The model under review builds one solid part; all positions refer to its coordinate system, in mm. A direction names the side the tool comes from. Give positions to 0.01 mm unless a question says otherwise; leave off trailing zeros. Loops run counter-clockwise (first coordinate to the right, second up) from the corner with the lowest first, then second, coordinate; pieces in that order, holes last. Notation, with made-up numbers: M -17.5,-24.75 L 1.5,-24.75 A21 ccw 1.5,-8.75 Z; hole C 71,-16.75 d7. An arc over 180 degrees is marked long. Write item = value, one per line. Start each with the question number.
1. We need section C-C on x = 60.5. Give the boundary of the cut face in (y, z).
2. Wall thickness on line 1 along Y through (x, z) = (37, -63); line 2 along Z through (x, y) = (17, 10); line 3 along Z through (x, y) = (38, 7.25): over which ranges is each line inside the solid? List them lowest first. Write a range as from..to.
3. For faces 5 (the face through (34.194, 2.465, -49.688)), 6 (the face through (46, 0, -1)), 7 (the face through (22.761, 17.521, 51.585)), list the 3-axis set-ups (+Z, -Z, +X, -X, +Y, -Y) from which the entire face can be reached by the end or side of a thin tool; tool diameter is ignored.
4. For pin 1 (1 mm diameter, centred on x = 54, y = 12, fed in from +Z); pin 2 (6 mm diameter, centred on y = 16.5, z = -31.5, fed in from +X); pin 3 (9 mm diameter, centred on y = 10, z = -63, fed in from +X); pin 4 (8 mm diameter, centred on x = 30.82, z = 53.37, fed in from -Y), all flat-tipped, find the tip position at first contact; note any pin that passes through.
5. We need section A-A on y = 7.5. Give the boundary of the cut face in (x, z) (3 decimals).
6. Draft analysis for pull direction X (two halves, no side actions). For faces 1 (the face through (33, 16, 51)), 2 (the face through (46, 20, -1)), 3 (the face through (29, 5, 51)), 4 (the face through (74.98, 9.86, -1.65)), state which applies: pulls with the +X half, pulls with the -X half, needs draft (parallel to the pull), parting line crosses it, or undercut.
7. We need section B-B on z = 0. Give the boundary of the cut face in (x, y), then the cut area to 3 significant figures.
from build123d import *

# Parameters (mm, degrees)
BOSS_EXTRUDE1_DEPTH = 20
SKETCH2_R           = 5
CUT_EXTRUDE1_DEPTH  = 150
SKETCH3_R           = 8.25
CUT_EXTRUDE3_DEPTH  = 4
SKETCH4_R           = 2.75
CUT_EXTRUDE4_DEPTH  = 20
SKETCH5_R           = 5
CUT_EXTRUDE5_DEPTH  = 5
FILLET1_R           = 1


with BuildPart() as part:
    # Sketch1 → Boss-Extrude1 (new body)
    with BuildSketch(Plane(origin=(0, 0, 0), x_dir=(1, 0, 0), z_dir=(0, 1, 0))):
        with BuildLine():
            Line((0, 44.25), (0, 75))
            ThreePointArc((0, 75), (75, 0), (0, -75))
            Line((0, -75), (0, -44.25))
            ThreePointArc((0, -44.25), (44.25, 0), (0, 44.25))
        make_face()
    extrude(amount=BOSS_EXTRUDE1_DEPTH)

    # Sketch2 → Cut-Extrude1 (cut)
    with BuildSketch(Plane.ZY):
        with Locations((-63, 10)):
            Circle(SKETCH2_R)
        with Locations((63, 10)):
            Circle(SKETCH2_R)
    extrude(amount=-CUT_EXTRUDE1_DEPTH, mode=Mode.SUBTRACT)

    # Sketch3 → Cut-Extrude3 (cut)
    with BuildSketch(Plane(origin=(0, 20, 0), x_dir=(1, 0, 0), z_dir=(0, 1, 0))):
        with Locations(Location((30.815, -53.373145635, 0), (0, 0, 270))):
            Circle(SKETCH3_R)
        with Locations(Location((30.815, 53.373145635, 0), (0, 0, 270))):
            Circle(SKETCH3_R)
    extrude(amount=-CUT_EXTRUDE3_DEPTH, mode=Mode.SUBTRACT)

    # Sketch4 → Cut-Extrude4 (cut)
    with BuildSketch(Plane(origin=(0, 16, 0), x_dir=(1, 0, 0), z_dir=(0, 1, 0))):
        with Locations(Location((30.815, 53.373145635, 0), (0, 0, 270))):
            Circle(SKETCH4_R)
        with Locations(Location((30.815, -53.373145635, 0), (0, 0, 270))):
            Circle(SKETCH4_R)
    extrude(amount=-CUT_EXTRUDE4_DEPTH, mode=Mode.SUBTRACT)

    # Sketch5 → Cut-Extrude5 (cut)
    with BuildSketch(Plane.XZ):
        with Locations(Location((30.815, 53.373145635, 0), (0, 0, 270))):
            Circle(SKETCH5_R)
        with Locations(Location((30.815, -53.373145635, 0), (0, 0, 270))):
            Circle(SKETCH5_R)
    extrude(amount=-CUT_EXTRUDE5_DEPTH, mode=Mode.SUBTRACT)

    # Fillet1
    fillet1_edges = [part.edges().sort_by_distance(p)[0] for p in [
        (30.815, 20, 45.123145635),
        (30.815, 20, -61.623145635),
    ]]
    fillet(fillet1_edges, radius=FILLET1_R)


solid = part.part
Final values:
q1.outline = M 0,-44.33 L 20,-44.33 L 20,44.33 L 0,44.33 Z
q2.line_1 = 0..5, 15..20
q2.line_2 = -73.05..-68, -58..-40.85, 40.85..58, 68..73.05
q2.line_3 = -58.82..-22.67, 22.67..58.82
q3.face_5 = -Y
q3.face_6 = +Z, -Z, +X, -X, -Y
q3.face_7 = +Y
q4.pin_1 = 52.56
q4.pin_2 = 69.37
q4.pin_3 = through
q4.pin_4 = 5
q5.outline = M 0,-75 A75 ccw 33.04,-67.33 L 0,-67.33 Z; M 0,-58.67 L 46.721,-58.67 A75 ccw 46.721,58.67 L 0,58.67 L 0,44.25 A44.25 cw 0,-44.25 Z; M 0,67.33 L 33.04,67.33 A75 ccw 0,75 Z; hole C 30.815,-53.373 d5.5; hole C 30.815,53.373 d5.5
q6.face_1 = undercut
q6.face_2 = needs draft
q6.face_3 = undercut
q6.face_4 = pulls with the +X half
q7.outline = M 44.25,0 L 75,0 L 75,20 L 44.25,20 Z
q7.area = 615 mm²
